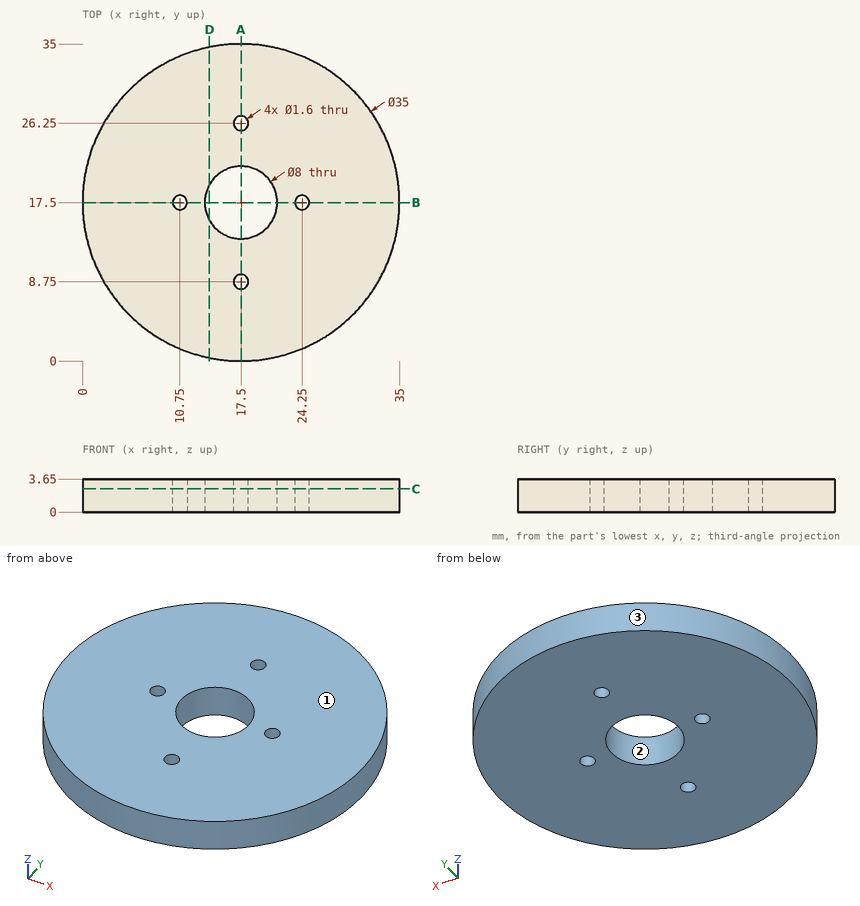
Verification items for this drawing (mm, ordinates from the low corner). Round coordinates to 2 decimals unless told otherwise and drop trailing zeros. Write each loop counter-clockwise with the first axis right and the second up, starting at its lowest first coordinate (ties: lowest second). Pieces come first, ordered by that corner, then holes. Notation, with made-up numbers: (57.25, 85.25) - (63.25, 85.25) arc R16 cw to (63.25, 99.25) - close; hole circle Ø1 at (-19, 55.5). An arc over 180 degrees is marked (long way). One line per item, written item: value.
1. Cross-section at C-C on z = 2.55. Record the boundary of the cut face in (x, y), and give its area (3 significant figures).
The answers:
outline: circle Ø35 at (17.5, 17.5); hole circle Ø1.6 at (10.75, 17.5); hole circle Ø8 at (17.5, 17.5); hole circle Ø1.6 at (17.5, 8.75); hole circle Ø1.6 at (17.5, 26.25); hole circle Ø1.6 at (24.25, 17.5)
area: 904 mm^2
2. Cross-section at D-D on x = 14. Record the boundary of the cut face in (y, z).
The answers:
outline: (0.35, 0) - (15.56, 0) - (15.56, 3.65) - (0.35, 3.65) - close; (19.44, 0) - (34.65, 0) - (34.65, 3.65) - (19.44, 3.65) - close
3. Mould release check, pull along Y, two halves, no side actions. Record for the marked faces 1, 2 and 3: released by +Y, released by -Y, zero draft, split by the parting line, or undercut.
The answers:
face 1: zero draft
face 2: undercut
face 3: split by the parting line
4. Cross-section at A-A on x = 17.5. Record the boundary of the cut face in (y, z).
The answers:
outline: (0, 0) - (7.95, 0) - (7.95, 3.65) - (0, 3.65) - close; (9.55, 0) - (13.5, 0) - (13.5, 3.65) - (9.55, 3.65) - close; (21.5, 0) - (25.45, 0) - (25.45, 3.65) - (21.5, 3.65) - close; (27.05, 0) - (35, 0) - (35, 3.65) - (27.05, 3.65) - close
5. Scan lines: L1, parallel to Y at x = 17.5, z = 2.45; L2, parallel to Y at x = 18, z = 0.6; L3, parallel to X at y = 19, z = 3. Record each from-to range of solid material in increasing order.
The answers:
L1: y = 0 to 7.95, 9.55 to 13.5, 21.5 to 25.45, 27.05 to 35
L2: y = 0.01 to 8.13, 9.37 to 13.53, 21.47 to 25.63, 26.87 to 34.99
L3: x = 0.06 to 13.79, 21.21 to 34.94
6. Cross-section at B-B on y = 17.5. Record the boundary of the cut face in (x, z), and give its area (3 significant figures).
The answers:
outline: (0, 0) - (9.95, 0) - (9.95, 3.65) - (0, 3.65) - close; (11.55, 0) - (13.5, 0) - (13.5, 3.65) - (11.55, 3.65) - close; (21.5, 0) - (23.45, 0) - (23.45, 3.65) - (21.5, 3.65) - close; (25.05, 0) - (35, 0) - (35, 3.65) - (25.05, 3.65) - close
area: 86.9 mm^2
7. Depth check by flat-ended pin: pin 1 Ø2 at (x, y) = (17.5, 26.25) entering from +Z; pin 2 Ø1.4 at (x, y) = (24.25, 17.5) entering from -Z; pin 3 Ø2 at (y, z) = (29.5, 0.5) entering from +X; pin 4 Ø1 at (y, z) = (10, 2.5) entering from -X. Enter the tip coordinate at first touch or a pass-through.
The answers:
pin 1: stops at z = 3.65
pin 2: passes through
pin 3: stops at x = 31.11
pin 4: stops at x = 1.46
